Source: CAD feature listing. Evaluate the final solid. Frame: model axes, mm. A direction names the side the tool comes from. Coordinates: 2 decimals unless noted, no trailing zeros. Write each loop counter-clockwise with the first axis right and the second up, starting at its lowest first coordinate (ties: lowest second). Pieces come first, ordered by that corner, then holes. Notation, with made-up numbers: (31, -4) - (57, -4) arc R10 ccw to (57, 7) - close; hole circle Ø3 at (-3.75, -22.75). An arc over 180 degrees is marked (long way). One line per item, written item: value.
from build123d import *

# Parameters (mm, degrees)
F0_W     = 10
F0_H     = 10
F1_DEPTH = 5
F2_W     = 4
F2_H     = 4
F3_DEPTH = 15
F4_W     = 4
F4_H     = 4
F5_DEPTH = 15
F6_W     = 4
F6_H     = 4
F7_DEPTH = 15
F8_DEPTH = 15


with BuildPart() as f1:
    # F0 (on Top) → F1 (new body, symmetric)
    with BuildSketch(Plane.XY):
        Rectangle(F0_W, F0_H)
    extrude(amount=F1_DEPTH, both=True)

    # F2 (on Top) → F3 (join)
    with BuildSketch(Plane.XY):
        Rectangle(F2_W, F2_H)
    extrude(amount=F3_DEPTH)

    # F4 (on Front) → F5 (join)
    with BuildSketch(Plane.XZ):
        Rectangle(F4_W, F4_H)
    extrude(amount=F5_DEPTH)

    # F6 (on Right) → F7 (join)
    with BuildSketch(Plane.YZ):
        Rectangle(F6_W, F6_H)
    extrude(amount=F7_DEPTH)

    # F6 (on Right) → F8 (join)
    with BuildSketch(Plane.YZ):
        Rectangle(F6_W, F6_H)
    extrude(amount=-F8_DEPTH)


solid = f1.part
1) Material intervals for line 1 (Y direction, x = 1.25, z = -3); line 2 (Z direction, x = -10, y = -0.5), sorted ascending.
Values found:
line 1: -5 to 5
line 2: -2 to 2
2) Section query D-D on y = -5.75. Output: boundary loops of the cut face in (x, z).
Values found:
outline: (-2, -2) - (2, -2) - (2, 2) - (-2, 2) - close
3) Section query B-B on y = -1.25. Output: boundary loops of the cut face in (x, z).
Values found:
outline: (-15, -2) - (-5, -2) - (-5, -5) - (5, -5) - (5, -2) - (15, -2) - (15, 2) - (5, 2) - (5, 5) - (2, 5) - (2, 15) - (-2, 15) - (-2, 5) - (-5, 5) - (-5, 2) - (-15, 2) - close
4) Reachability of faces 1 (the flat face through (-10, 0, -2)), 2 (the flat face through (2, 0, 10)), 3 (the flat face through (2, -10, 0)), 4 (the flat face through (-2, -10, 0)), 5 (the flat face through (0, 2, 10)) from +Z, -Z, +X, -X, +Y, -Y: full face, straight path, thin tool, end or side. Return the list, or none.
Values found:
face 1: -Z, -X, +Y, -Y
face 2: +Z, +X, +Y, -Y
face 3: +Z, -Z, +X, -Y
face 4: +Z, -Z, -X, -Y
face 5: +Z, +X, -X, +Y
5) Section query C-C on x = 4.25. Output: boundary loops of the cut face in (y, z), then the cut area to 3 significant figures.
Values found:
outline: (-5, -5) - (5, -5) - (5, 5) - (-5, 5) - close
area: 100 mm2
6) Section query A-A on z = 1.5. Output: boundary loops of the cut face in (x, y), then the cut area to 3 significant figures.
Values found:
outline: (-15, -2) - (-5, -2) - (-5, -5) - (-2, -5) - (-2, -15) - (2, -15) - (2, -5) - (5, -5) - (5, -2) - (15, -2) - (15, 2) - (5, 2) - (5, 5) - (-5, 5) - (-5, 2) - (-15, 2) - close
area: 220 mm2
7) Contact query for flat-ended pins moving along their axis: P1, Ø5, axis at x = -1, z = 2.5, coming from the -Y side; P2, Ø4, axis at y = -6.5, z = 0.5, coming from the -X side; P3, Ø2, axis at y = -12.5, z = -1, coming from the +X side; P4, Ø4.5, axis at x = 8, z = 0.5, coming from the +Y side. Output: stop coordinate, or through.
Values found:
P1: y = -15
P2: x = -5
P3: x = 2
P4: y = 2
